Check sheet for the drawn part. Datum: minimum x, y, z corner. Units: mm. A direction names the side the tool comes from. Round coordinates to 2 decimals unless told otherwise and drop trailing zeros. Write each loop counter-clockwise with the first axis right and the second up, starting at its lowest first coordinate (ties: lowest second). Pieces come first, ordered by that corner, then holes. Notation, with made-up numbers: (56, -13) - (62, -13) arc R24 ccw to (62, 17) - close; hole circle Ø2 at (85, 65.25). An arc over 180 degrees is marked (long way). Answer as a JSON object with one key per item and string values.
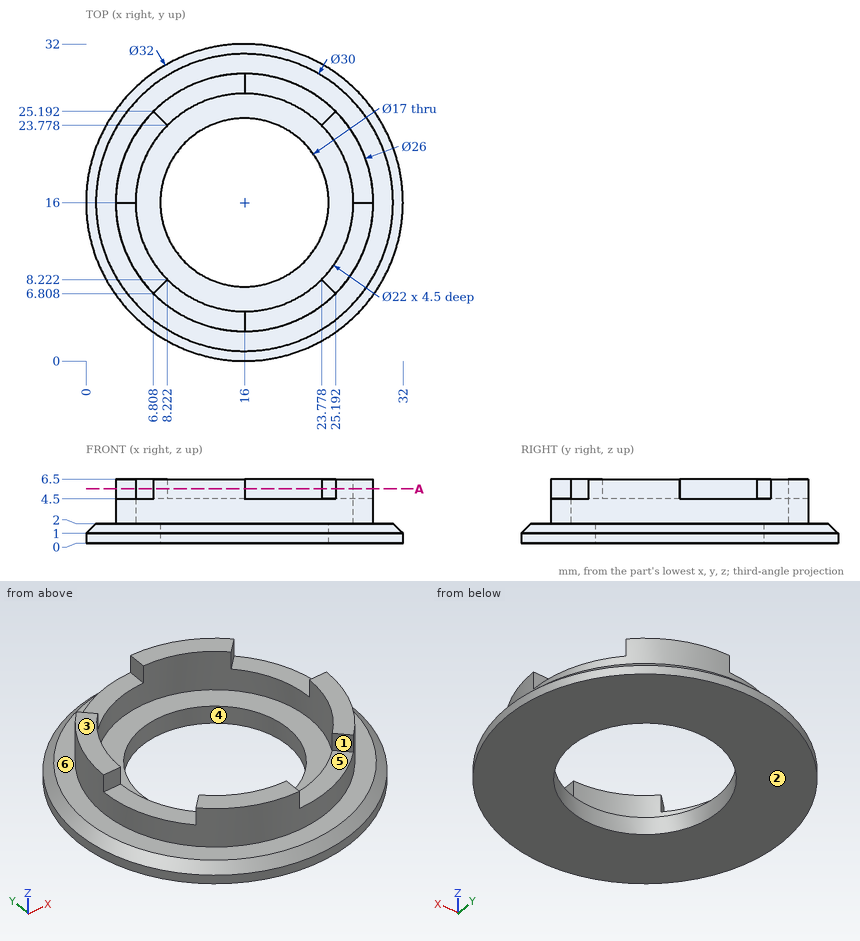
Q1. Release check for a two-part mould opening along Z. For the marked faces 1, 2 and 3 record: released by +Z, released by -Z, zero draft, split by the parting line, or undercut.
Geometry check:
{"face 1": "zero draft", "face 2": "released by -Z", "face 3": "released by +Z"}
Q2. Material ranges on line 1 along Y through (x, z) = (16, 3.25); line 2 along Y through (x, z) = (12.5, 4.25), recorded low to high. Write a range as [from, to].
Geometry check:
{"line 1": "y = [3, 5], [27, 29]", "line 2": "y = [3.48, 5.57], [26.43, 28.52]"}
Q3. Section check A-A, the plane z = 5.5. Record the cut outline in (x, y).
Geometry check:
{"outline": "(3, 16) - (5, 16) arc R11 cw to (8.22, 23.78) - (6.81, 25.19) arc R13 ccw to start; (6.81, 6.81) arc R13 ccw to (16, 3) - (16, 5) arc R11 cw to (8.22, 8.22) - close; (16, 27) arc R11 cw to (23.78, 23.78) - (25.19, 25.19) arc R13 ccw to (16, 29) - close; (23.78, 8.22) - (25.19, 6.81) arc R13 ccw to (29, 16) - (27, 16) arc R11 cw to start"}
Q4. Gauge pin test, flat ends, axial feed: P1, Ø4, axis at x = 19, y = 25, coming from the -Z side; P2, Ø1, axis at x = 5.5, z = 1, coming from the +Y side; P3, Ø3, axis at y = 6, z = 1, coming from the -X side (1 decimal); P4, Ø6.5, axis at x = 12, y = 20, coming from the +Z side. Record the tip position at first contact, or that the pin passes through.
Geometry check:
{"P1": "stops at z = 0", "P2": "stops at y = 28.49", "P3": "stops at x = 2.4", "P4": "stops at z = 2"}
Q5. Set-up check for the marked faces 4, 5 and 6: record each of +Z, -Z, +X, -X, +Y, -Y from which the full face is reachable in a straight line by a thin tool's end or side.
Geometry check:
{"face 4": "+Z, -Z", "face 5": "+Z, -Y", "face 6": "+Z"}
